The model under review builds one solid part; all positions refer to its coordinate system, in mm. A direction names the side the tool comes from. Round coordinates to 2 decimals unless told otherwise and drop trailing zeros. Write each loop counter-clockwise with the first axis right and the second up, starting at its lowest first coordinate (ties: lowest second). Pieces come first, ordered by that corner, then holes. Notation, with made-up numbers: (62, 69) - (83, 69) arc R28 ccw to (83, 92) - close; hole circle Ø11 at (73.25, 87). An arc over 180 degrees is marked (long way). Use one line per item in the form item = value.
from build123d import *

# Parameters (mm, degrees)
SKETCH1_R           = 40
BOSS_EXTRUDE1_DEPTH = 10
SKETCH2_R           = 10
BOSS_EXTRUDE2_DEPTH = 10
SKETCH3_R           = 5
CUT_EXTRUDE1_DEPTH  = 20
SKETCH4_R           = 1.65
CUT_EXTRUDE2_DEPTH  = 10


with BuildPart() as part:
    # Sketch1 → Boss-Extrude1 (new body)
    with BuildSketch(Plane.XY):
        Circle(SKETCH1_R)
    extrude(amount=BOSS_EXTRUDE1_DEPTH)

    # Sketch2 → Boss-Extrude2 (add)
    with BuildSketch(Plane.XY.offset(10)):
        Circle(SKETCH2_R)
    extrude(amount=BOSS_EXTRUDE2_DEPTH)

    # Sketch3 → Cut-Extrude1 (cut)
    with BuildSketch(Plane.XY):
        Circle(SKETCH3_R)
    extrude(amount=CUT_EXTRUDE1_DEPTH, mode=Mode.SUBTRACT)

    # Sketch4 → Cut-Extrude2 (cut)
    with BuildSketch(Plane(origin=(0, 0, 0), x_dir=(1, 0, 0), z_dir=(0, 1, 0))):
        with Locations(Location((0, -15, 0), (0, 0, 90))):
            Circle(SKETCH4_R)
    extrude(amount=CUT_EXTRUDE2_DEPTH, mode=Mode.SUBTRACT)


solid = part.part
(1) Add section D-D on y = 8. Write out the cut boundary in (x, z).
Geometry results:
outline = (-39.19, 0) - (39.19, 0) - (39.19, 10) - (6, 10) - (6, 20) - (-6, 20) - (-6, 10) - (-39.19, 10) - close; hole circle Ø3.3 at (0, 15)
(2) Machinability: for faces 4 (the cylindrical face through (-2.17, -9.76, 14.93)), 5 (the flat face through (-5, -2, 20)), 6 (the cylindrical face through (0.632, 7.323, 13.476)), which of the approach directions +Z, -Z, +X, -X, +Y, -Y give a long, thin tool a straight path to every point of the face, cutting with its end or side? Answer none if there is none.
Geometry results:
face_4 = +Z
face_5 = +Z, +X, -X, +Y, -Y
face_6 = +Y
(3) Add section A-A on x = 0. Write out the cut boundary in (y, z).
Geometry results:
outline = (-40, 0) - (-5, 0) - (-5, 20) - (-10, 20) - (-10, 10) - (-40, 10) - close; (5, 0) - (40, 0) - (40, 10) - (10, 10) - (10, 13.35) - (5, 13.35) - close; (5, 16.65) - (10, 16.65) - (10, 20) - (5, 20) - close
(4) Add section B-B on y = 0. Write out the cut boundary in (x, z).
Geometry results:
outline = (-40, 0) - (-5, 0) - (-5, 20) - (-10, 20) - (-10, 10) - (-40, 10) - close; (5, 0) - (40, 0) - (40, 10) - (10, 10) - (10, 20) - (5, 20) - close
(5) Insertion check: P1, Ø8, axis at x = 21.5, z = 5.5, coming from the -Y side; P2, Ø10, axis at y = -8.5, z = 6, coming from the -X side; P3, Ø10, axis at x = -8, y = -30.5, coming from the +Z side. Each pin has a flat end and moves straight along its axis. Give the tip position at first contact, or say it passes through.
Geometry results:
P1 = -35.97
P2 = -39.85
P3 = 10
(6) To check wall thickness, follow L1, parallel to Y at x = 0, z = 7.5; L2, parallel to Z at x = 23, y = -30; L3, parallel to X at y = 6.35, z = 15. State the ranges of each line that lie inside material, in increasing order.
Geometry results:
L1 = -40 to -5, 5 to 40
L2 = 0 to 10
L3 = -7.73 to -1.65, 1.65 to 7.73
(7) The part is to be moulded in two halves that separate along Y. For faces 1 (the cylindrical face through (-1.08, -4.88, 9.86)), 2 (the flat face through (8, -8, 10)), 3 (the cylindrical face through (-8.67, -39.05, 4.93)), say which applies: +Y half, -Y half, draft (parallel to the pull), parting line (faces both ways), or undercut.
Geometry results:
face_1 = undercut
face_2 = draft
face_3 = parting line
(8) Add section C-C on z = 17.75. Write out the cut boundary in (x, y), then the cut area to 3 significant figures.
Geometry results:
outline = circle Ø20 at (0, 0); hole circle Ø10 at (0, 0)
area = 236 mm2
